Study the drawing (mm; zero at the part's minimum x, y, z) and answer. A direction names the side the tool comes from. Coordinates: 2 decimals unless noted, no trailing zeros. Order: outer loops, then holes, each group sorted by start corner. A loop starts at its lowest first (then second) coordinate and runs counter-clockwise, first axis right, second up. Notation, with made-up numbers: (-39.75, -38.75) -> (-2.75, -38.75) arc R16 ccw to (-2.75, -30.75) -> close; hole circle Ø5 at (89.5, 77.25). An arc over 180 degrees is marked (long way). Put each result on its own line as item: value. Start each with the question number.
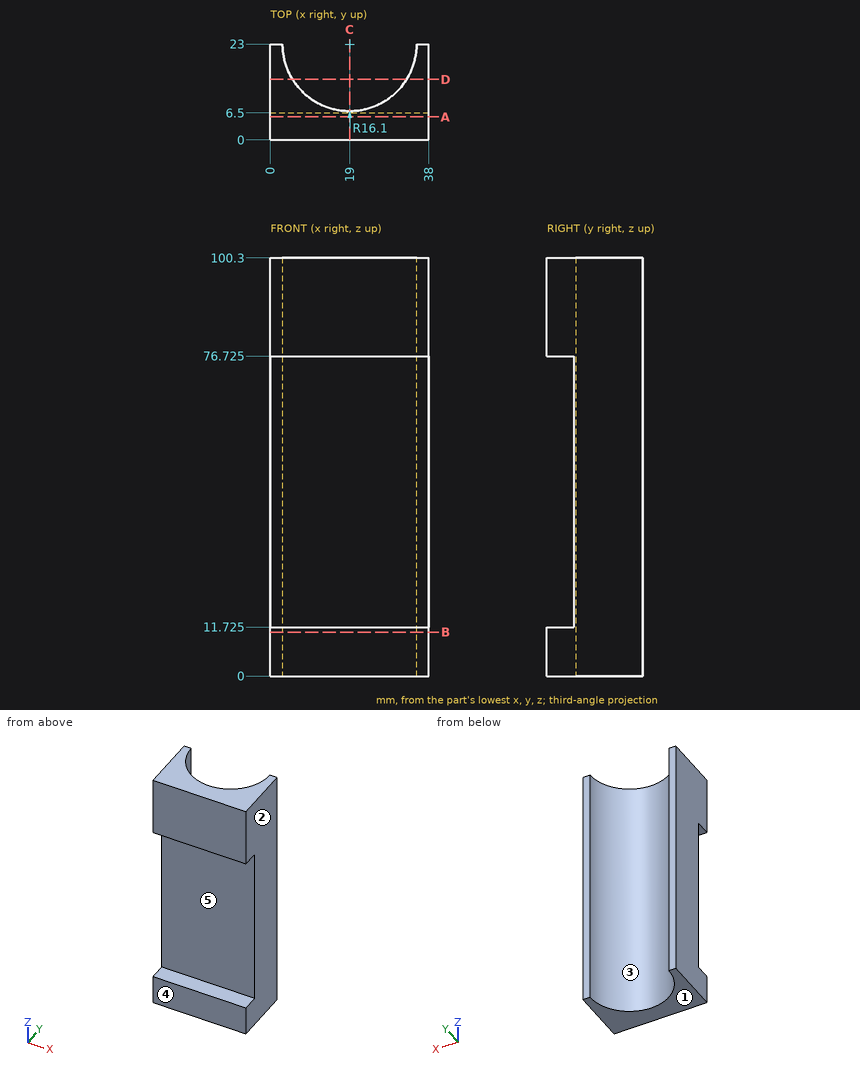
(1) A tool of negligible diameter and unlimited length cuts with its end or side. For the marked faces 4 and 5, from which of +Z, -Z, +X, -X, +Y, -Y can it reach the whole face along a straight path? Write none if from no direction.
(2) Find the intervals of material crossed by L1, parallel to Z at x = 27, y = 4.25 (3 decimals); L2, parallel to X at y = 12, z = 63; L3, parallel to X at y = 17, z = 13, in increasing order.
(3) The part is cut by section D-D on y = 14.5. Determine the outline of the cut face in (x, z).
(4) The part is cut by section C-C on x = 19. Determine the outline of the cut face in (y, z) (3 decimals), plus the area to 3 significant figures.
(5) The part is cut by section A-A on y = 5.5. Determine the outline of the cut face in (x, z) (3 decimals).
(6) Each of these flat-tipped pins is pushed along its axis until it touches: P1, Ø19, axis at x = 13.5, z = 55, coming from the -Y side; P2, Ø4, axis at x = 21.5, z = 17, coming from the +Y side. Where does it stop, or does it pass through?
(7) The part is cut by section B-B on z = 10.5. Determine the outline of the cut face in (x, y), plus the area to 3 significant figures.
(8) For a pull along X with two mould halves and no side action, classify the marked faces 1, 2 and 3 as released by +X, released by -X, zero draft, split by the parting line, or undercut.
Worked out:
1. face 4: +Z, -Z, +X, -X, -Y
1. face 5: +X, -X, -Y
2. L1: 0 to 11.725, 76.725 to 100.3
2. L2: 0 to 7.24, 30.76 to 38
2. L3: 0 to 4.06, 33.94 to 38
3. outline: (0, 0) -> (5.33, 0) -> (5.33, 100.3) -> (0, 100.3) -> close; (32.67, 0) -> (38, 0) -> (38, 100.3) -> (32.67, 100.3) -> close
4. outline: (0, 0) -> (6.9, 0) -> (6.9, 100.3) -> (0, 100.3) -> (0, 76.725) -> (6.5, 76.725) -> (6.5, 11.725) -> (0, 11.725) -> close
4. area: 270 mm2
5. outline: (0, 0) -> (38, 0) -> (38, 11.725) -> (0, 11.725) -> close; (0, 76.725) -> (38, 76.725) -> (38, 100.3) -> (0, 100.3) -> close
6. P1: y = 6.5
6. P2: y = 7.54
7. outline: (0, 0) -> (38, 0) -> (38, 23) -> (35.1, 23) arc R16.1 cw to (2.9, 23) -> (0, 23) -> close
7. area: 467 mm2
8. face 1: zero draft
8. face 2: released by +X
8. face 3: undercut
